from build123d import *

# Parameters (mm, degrees)
SKETCH1_R           = 13.9065
BOSS_EXTRUDE1_DEPTH = 14.9225
SKETCH2_R           = 13.9065
SKETCH2_R_2         = 4.4958
CUT_EXTRUDE1_DEPTH  = 3.937
SKETCH3_W           = 6.985
SKETCH3_H           = 3.175
BOSS_EXTRUDE2_DEPTH = 25.4
SKETCH4_R           = 1.5
CUT_EXTRUDE2_DEPTH  = 12.7


with BuildPart() as part:
    # Sketch1 → Boss-Extrude1 (new body, symmetric)
    with BuildSketch(Plane(origin=(0, 0, 0), x_dir=(1, 0, 0), z_dir=(0, 1, 0))):
        Circle(SKETCH1_R)
    extrude(amount=BOSS_EXTRUDE1_DEPTH, both=True)

    # Sketch2 → Cut-Extrude1 (cut)
    with BuildSketch(Plane(origin=(0, 14.9225, 0), x_dir=(1, 0, 0), z_dir=(0, 1, 0))):
        Circle(SKETCH2_R)
        Circle(SKETCH2_R_2, mode=Mode.SUBTRACT)
    extrude(amount=-CUT_EXTRUDE1_DEPTH, mode=Mode.SUBTRACT)

    # Sketch3 → Boss-Extrude2 (add)
    with BuildSketch(Plane.XY):
        with Locations((0, -10.795)):
            Rectangle(SKETCH3_W, SKETCH3_H)
    extrude(amount=BOSS_EXTRUDE2_DEPTH)

    # Sketch4 → Cut-Extrude2 (cut)
    with BuildSketch(Plane.XZ.offset(14.9225)):
        with Locations((-5.656854249, 5.656854249)):
            Circle(SKETCH4_R)
        with Locations((6.717514421, 6.717514421)):
            Circle(SKETCH4_R)
        with Locations((5.656854249, -5.656854249)):
            Circle(SKETCH4_R)
        with Locations((-6.717514421, -6.717514421)):
            Circle(SKETCH4_R)
    extrude(amount=-CUT_EXTRUDE2_DEPTH, mode=Mode.SUBTRACT)


solid = part.part
Geometry: final body of the model. Coordinates: model frame, mm. A direction names the side the tool comes from. Round coordinates to 2 decimals unless told otherwise and drop trailing zeros. Order: outer loops, then holes, each group sorted by start corner. A loop starts at its lowest first (then second) coordinate and runs counter-clockwise, first axis right, second up.
Q1. Section A-A, the plane y = -10.5. Output: boundary loops of the cut face in (x, z).
Result sheet:
outline: (-3.49, 13.46) arc R13.91 ccw (long way) to (3.49, 13.46) - (3.49, 25.4) - (-3.49, 25.4) - close; hole circle Ø3 at (-6.72, -6.72); hole circle Ø3 at (-5.66, 5.66); hole circle Ø3 at (5.66, -5.66); hole circle Ø3 at (6.72, 6.72)
Q2. Material intervals for probe 1 along X at (y, z) = (-5.75, 6); probe 2 along X at (y, z) = (-5.25, -7); probe 3 along Y at (x, z) = (-12.25, 0), sorted ascending.
Result sheet:
probe 1: x = -12.55 to -7.12, -4.2 to 5.4, 8.03 to 12.55
probe 2: x = -12.02 to -8.19, -5.24 to 4.99, 6.32 to 12.02
probe 3: y = -14.92 to 10.99
Q3. Section C-C, the plane z = 0. Output: boundary loops of the cut face in (x, y).
Result sheet:
outline: (-13.91, -14.92) - (13.91, -14.92) - (13.91, 10.99) - (4.5, 10.99) - (4.5, 14.92) - (-4.5, 14.92) - (-4.5, 10.99) - (-13.91, 10.99) - close
Q4. Section B-B, the plane x = 0. Output: boundary loops of the cut face in (y, z), and give its area (3 significant figures).
Result sheet:
outline: (-14.92, -13.91) - (10.99, -13.91) - (10.99, -4.5) - (14.92, -4.5) - (14.92, 4.5) - (10.99, 4.5) - (10.99, 13.91) - (-9.21, 13.91) - (-9.21, 25.4) - (-12.38, 25.4) - (-12.38, 13.91) - (-14.92, 13.91) - close
area: 792 mm2
Q5. Section D-D, the plane y = 9.5. Output: boundary loops of the cut face in (x, z).
Result sheet:
outline: circle Ø27.81 at (0, 0)
Q6. Pin query (flat end, axial travel): pin 1 (2.5 mm diameter, centred on x = -5.66, z = 5.66, fed in from +Y); pin 2 (1.8 mm diameter, centred on x = 6.72, z = 6.72, fed in from -Y); pin 3 (7.5 mm diameter, centred on x = 1.5, z = 21.5, fed in from -Y); pin 4 (5 mm diameter, centred on x = 11, z = 13, fed in from -Y). Return the tip coordinate at first contact, or that it passes through.
Result sheet:
pin 1: stops at y = 10.99
pin 2: stops at y = -2.22
pin 3: stops at y = -12.38
pin 4: passes through
Q7. Access query for faces 1 (the face through (-3.492, -11, 19)), 2 (the face through (-3.3, 10.986, -3.3)), 3 (the face through (6, -2.222, -6)). Directions: +Z, -Z, +X, -X, +Y, -Y. A direction counts if a zero-diameter tool reaches every point of the face in a straight line with its end or side. Return the directions, or none.
Result sheet:
face 1: +Z, -X, +Y, -Y
face 2: +Y
face 3: -Y
Q8. Mould query, pull axis X, two halves, no side actions, for faces 4 (the face through (0, -12.382, 19)), 5 (the face through (8.148, -8.661, 7.168)), 6 (the face through (4.153, 12.982, 1.722)). Classes: released by +X, released by -X, zero draft, split by the parting line, or undercut.
Result sheet:
face 4: zero draft
face 5: undercut
face 6: split by the parting line
